For this review, take the finished solid that the model builds, in its own axes (mm). A direction names the side the tool comes from. Give positions to 0.01 mm unless a question says otherwise; leave off trailing zeros. Loops run counter-clockwise (first coordinate to the right, second up) from the corner with the lowest first, then second, coordinate; pieces in that order, holes last.
```python
from build123d import *

# Parameters (mm, degrees)
CHAMFER1_SIZE       = 0.254
CUT_EXTRUDE3_DEPTH  = 3.81
SKETCH5_R           = 0.9525
BOSS_EXTRUDE1_DEPTH = 3.7592
CUT_EXTRUDE1_DEPTH  = 137.608260621
CHAMFER2_SIZE       = 0.127
CUT_EXTRUDE4_REACH  = 83.566
FILLET1_R           = 0.508
FILLET2_R           = 0.127


with BuildPart() as part:
    # Sketch1 → Revolve1 (revolve)
    with BuildSketch(Plane.XY, mode=Mode.PRIVATE) as revolve1_sk:
        Polygon((0, 82.4738), (1.23825, 82.4738), (1.23825, 2.5908), (3.6322, 2.5908), (4.8768, 1.3462), (3.96875, 1.3462), (3.96875, 0.4572), (5.969, 0.4572), (5.969, 0), (2.9845, 0), (2.9845, -5.842), (1.23825, -5.842), (1.23825, -53.8734), (0, -53.8734), align=None)
    revolve(revolve1_sk.sketch.rotate(Axis((0, 82.4738, 0), (0, -1, 0)), 180), axis=Axis((0, 82.4738, 0), (0, -1, 0)))

    # Chamfer1
    chamfer1_edges = [part.edges().sort_by_distance(p)[0] for p in [
        (1.23825, -53.8734, 0),
    ]]
    chamfer(chamfer1_edges, length=CHAMFER1_SIZE)

    # Sketch4 → Cut-Extrude3 (cut)
    with BuildSketch(Plane.XZ.offset(5.842)):
        with BuildLine():
            Line((-2.794, 1.049192189), (-2.794, -1.049192189))
            ThreePointArc((-2.794, -1.049192189), (-2.9845, 0), (-2.794, 1.049192189))
        make_face()
        with BuildLine():
            Line((2.794, 1.049192189), (2.794, -1.049192189))
            ThreePointArc((2.794, -1.049192189), (2.9845, 0), (2.794, 1.049192189))
        make_face()
    extrude(amount=-CUT_EXTRUDE3_DEPTH, mode=Mode.SUBTRACT)

    # Sketch5 → Boss-Extrude1 (add, symmetric)
    with BuildSketch(Plane(origin=(0, 0, 0), x_dir=(0, 0, -1), z_dir=(1, 0, 0))):
        with Locations(Location((0, -3.81, 0), (0, 0, 180))):
            Circle(SKETCH5_R)
    extrude(amount=BOSS_EXTRUDE1_DEPTH, both=True)

    # Sketch2 → Cut-Extrude1 (cut, through all)
    with BuildSketch(Plane.XZ.offset(53.8734)):
        with BuildLine():
            Line((0.254, 0.508), (0.254, -0.508))
            ThreePointArc((0.254, -0.508), (0, -0.762), (-0.254, -0.508))
            Line((-0.254, -0.508), (-0.254, 0.508))
            ThreePointArc((-0.254, 0.508), (0, 0.762), (0.254, 0.508))
        make_face()
    extrude(amount=-CUT_EXTRUDE1_DEPTH, mode=Mode.SUBTRACT)

    # Chamfer2
    chamfer2_edges = [part.edges().sort_by_distance(p)[0] for p in [
        (0, -5.842, 2.9845),
        (1.23825, 82.4738, 0),
        (0, -5.842, -2.9845),
        (-3.7592, -3.81, -0.9525),
        (3.7592, -3.81, -0.9525),
    ]]
    chamfer(chamfer2_edges, length=CHAMFER2_SIZE)

    # Sketch6 → Cut-Extrude4 (cut, up to next)
    with BuildSketch(Plane.XZ.offset(-1.3462), mode=Mode.PRIVATE) as cut_extrude4_sk1:
        with BuildLine():
            Line((-3.937, -2.878056504), (-3.937, 2.878056504))
            ThreePointArc((-3.937, 2.878056504), (-4.8768, 0), (-3.937, -2.878056504))
        make_face()
    cut_extrude4_tool1 = extrude(cut_extrude4_sk1.sketch, amount=-CUT_EXTRUDE4_REACH, mode=Mode.PRIVATE) & part.part
    # Sketch6 → Cut-Extrude4 (cut, up to next)
    with BuildSketch(Plane.XZ.offset(-1.3462), mode=Mode.PRIVATE) as cut_extrude4_sk2:
        with BuildLine():
            Line((3.937, -2.878056504), (3.937, 2.878056504))
            ThreePointArc((3.937, 2.878056504), (4.8768, 0), (3.937, -2.878056504))
        make_face()
    cut_extrude4_tool2 = extrude(cut_extrude4_sk2.sketch, amount=-CUT_EXTRUDE4_REACH, mode=Mode.PRIVATE) & part.part
    add(cut_extrude4_tool1.solids().sort_by_distance((-4.316209, 1.3462, 0))[0], mode=Mode.SUBTRACT)
    add(cut_extrude4_tool2.solids().sort_by_distance((4.316209, 1.3462, 0))[0], mode=Mode.SUBTRACT)

    # Fillet1
    fillet1_edges = [part.edges().sort_by_distance(p)[0] for p in [
        (1.23825, -5.842, 0),
    ]]
    fillet(fillet1_edges, radius=FILLET1_R)

    # Sketch7 → Revolve2 (revolve)
    with BuildSketch(Plane.XY):
        Polygon((1.23825, 5.278763066), (1.23825, 2.5908), (1.397, 2.5908), (1.397, 5.0038), align=None)
    revolve(axis=Axis((0, 0, 0), (0, 1, 0)))

    # Fillet2
    fillet2_edges = [part.edges().sort_by_distance(p)[0] for p in [
        (-1.397, 2.5908, 0),
    ]]
    fillet(fillet2_edges, radius=FILLET2_R)


solid = part.part
```
Item 1: Take a section at A-A on y = -39. Give the boundary of the cut face in (x, z), and give its area (3 significant figures).
Answer:
outline: circle Ø2.48 at (0, 0); hole (-0.25, -0.51) arc R0.25 ccw to (0.25, -0.51) - (0.25, 0.51) arc R0.25 ccw to (-0.25, 0.51) - close
area: 4.10 mm2
Item 2: Tool access review of faces 4 (the cylindrical face through (-1.11, 3.88, 0.85)), 5 (the flat face through (1, 0.457, 4)), 6 (the flat face through (-0.3, 1.346, -4.2)), 7 (the flat face through (1, 1.346, 4)), 8 (the cylindrical face through (-1.18, -30.32, -0.37)): name each direction out of +Z, -Z, +X, -X, +Y, -Y from which nothing blocks a thin tool from reaching the whole face with its end or side.
Answer:
face 4: +Y
face 5: none
face 6: -Z
face 7: +Z
face 8: -Y
Item 3: For L1, parallel to Y at x = 1.25, z = -2; L2, parallel to Y at x = -0.25, z = -3.5; L3, parallel to Z at x = -0.5, y = 37, list the stretches that pass through material, from the lowest coordinate up.
Answer:
L1: y = -5.84 to 2.59
L2: y = 0 to 2.59
L3: z = -1.13 to 1.13
Item 4: Clearance check with flat-ended pins moving along their axes: pin 1 Ø1 at (y, z) = (43, 1) entering from -X; pin 2 Ø0.5 at (y, z) = (2, -0.5) entering from +X; pin 3 Ø5 at (x, z) = (4.5, -1) entering from -Y. State where each tip first meets the part, or that it passes through.
Answer:
pin 1: stops at x = -1.13
pin 2: stops at x = 3.94
pin 3: stops at y = -5.84
Item 5: The part is to be moulded in two halves that separate along Y. For faces 1 (the cylindrical face through (0.86, 0.895, 3.874)), 2 (the flat face through (-2, -5.842, 0)), 3 (the cylindrical face through (1.294, 0.225, 5.827)), say which applies: released by +Y, released by -Y, zero draft, split by the parting line, or undercut.
Answer:
face 1: undercut
face 2: released by -Y
face 3: zero draft
